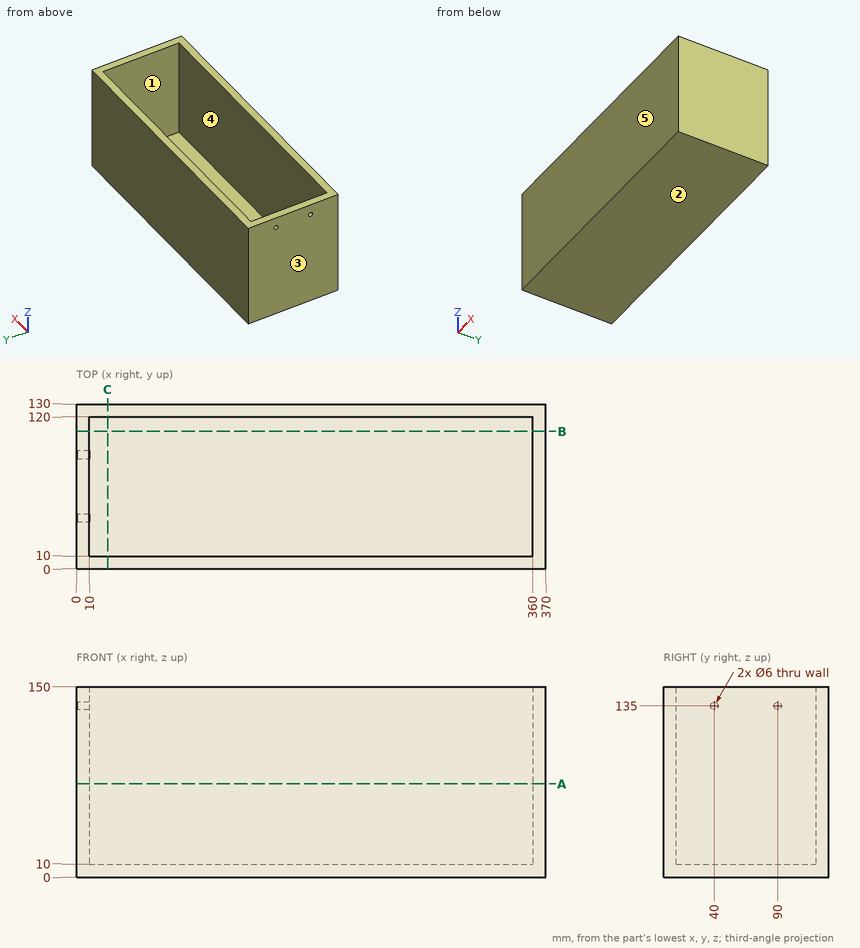
Geometry: see drawing. Coordinates: mm, zero at the bounding-box minimum. A direction names the side the tool comes from. Round coordinates to 2 decimals unless told otherwise and drop trailing zeros. Write each loop counter-clockwise with the first axis right and the second up, starting at its lowest first coordinate (ties: lowest second). Pieces come first, ordered by that corner, then holes.
1) Cut plane A-A (z = 73.5). Return the cut outline in (x, y).
2) Cut plane C-C (x = 24.5). Return the cut outline in (y, z).
3) Ray query, L1, parallel to Y at x = 5.25, z = 135; L2, parallel to X at y = 63, z = 40.5; L3, parallel to Z at x = 5.5, y = 90. Return the intervals inside material, ascending.
4) Draft query along Y for the marked faces 3, 4 and 5. Return one class per face: pulls with the +Y half, pulls with the -Y half, needs draft (parallel to the pull), parting line crosses it, or undercut.
5) Contact query for flat-ended pins moving along their axis: P1, Ø3.5, axis at y = 40, z = 135, coming from the -X side; P2, Ø1.5, axis at y = 46.5, z = 51.5, coming from the -X side. Output: stop coordinate, or through.
6) Cut plane B-B (y = 108.5). Return the cut outline in (x, z).
7) Reachability of the marked faces 1 and 2 from +Z, -Z, +X, -X, +Y, -Y: full face, straight path, thin tool, end or side. Return the list, or none.
Geometry says:
1. outline: (0, 0) - (370, 0) - (370, 130) - (0, 130) - close; hole (10, 10) - (360, 10) - (360, 120) - (10, 120) - close
2. outline: (0, 0) - (130, 0) - (130, 150) - (120, 150) - (120, 10) - (10, 10) - (10, 150) - (0, 150) - close
3. L1: y = 0 to 37, 43 to 87, 93 to 130
3. L2: x = 0 to 10, 360 to 370
3. L3: z = 0 to 132, 138 to 150
4. face 3: needs draft
4. face 4: undercut
4. face 5: pulls with the -Y half
5. P1: stops at x = 360
5. P2: stops at x = 0
6. outline: (0, 0) - (370, 0) - (370, 150) - (360, 150) - (360, 10) - (10, 10) - (10, 150) - (0, 150) - close
7. face 1: +Z
7. face 2: -Z, +X, -X, +Y, -Y
